Verification items for the finished model (mm, model axes). A direction names the side the tool comes from. Coordinates: 2 decimals unless noted, no trailing zeros. Write each loop counter-clockwise with the first axis right and the second up, starting at its lowest first coordinate (ties: lowest second). Pieces come first, ordered by that corner, then holes. Notation, with made-up numbers: (58, 48.5) -> (102, 48.5) arc R15 ccw to (102, 60.5) -> close; hole circle Ø4 at (20, 5.5). An arc over 180 degrees is marked (long way). Answer in a Markdown table with one row per item.
```python
from build123d import *

# Parameters (mm, degrees)
BOSS_EXTRUDE1_DEPTH = 10
SKETCH3_R           = 5
BOSS_EXTRUDE2_DEPTH = 5
SKETCH4_W           = 12.842437823
SKETCH4_H           = 1
CUT_EXTRUDE1_DEPTH  = 5
SKETCH5_R           = 3.418084762
BOSS_EXTRUDE3_DEPTH = 5
SKETCH6_W           = 9.346993936
SKETCH6_H           = 1
CUT_EXTRUDE2_DEPTH  = 5
SKETCH7_R           = 42.668113091
SKETCH7_R_2         = 32.812087574
BOSS_EXTRUDE4_DEPTH = 16
SKETCH8_R           = 10.204262611
CUT_EXTRUDE3_DEPTH  = 16
SKETCH9_R           = 41.320841223
SKETCH9_R_2         = 29.431774833
BOSS_EXTRUDE5_DEPTH = 16
SKETCH10_R          = 10.002103031
CUT_EXTRUDE4_DEPTH  = 16
SKETCH11_R          = 5.125485485
CUT_EXTRUDE5_DEPTH  = 16
SKETCH12_R          = 4.662079799
CUT_EXTRUDE6_DEPTH  = 16


with BuildPart() as part:
    # Sketch1 → Boss-Extrude1 (new body)
    with BuildSketch(Plane(origin=(0, 0, 0), x_dir=(1, 0, 0), z_dir=(0, 1, 0))):
        Polygon((0, 0), (0, 70), (-10, 70), (-10, -10), (70, -10), (70, 0), align=None)
    extrude(amount=BOSS_EXTRUDE1_DEPTH)

    # Sketch3 → Boss-Extrude2 (add)
    with BuildSketch(Plane.XY.offset(10)):
        with Locations((65, 5)):
            Circle(SKETCH3_R)
    extrude(amount=BOSS_EXTRUDE2_DEPTH)

    # Sketch4 → Cut-Extrude1 (cut)
    with BuildSketch(Plane.XY.offset(15)):
        with Locations((61.851491479, 5)):
            Rectangle(SKETCH4_W, SKETCH4_H)
    extrude(amount=-CUT_EXTRUDE1_DEPTH, mode=Mode.SUBTRACT)

    # Sketch5 → Boss-Extrude3 (add)
    with BuildSketch(Plane.ZY.offset(10)):
        with Locations(Location((-44.354632579, 5, 0), (0, 0, 180))):
            Circle(SKETCH5_R)
    extrude(amount=BOSS_EXTRUDE3_DEPTH)

    # Sketch6 → Cut-Extrude2 (cut)
    with BuildSketch(Plane.ZY.offset(15)):
        with Locations((-49.962828941, 2.5)):
            Rectangle(SKETCH6_W, SKETCH6_H)
    extrude(amount=-CUT_EXTRUDE2_DEPTH, mode=Mode.SUBTRACT)

    # Sketch7 → Boss-Extrude4 (add)
    with BuildSketch(Plane(origin=(0, 0, 0), x_dir=(-1, 0, 0), z_dir=(0, 0, -1))):
        with Locations((-70, 5)):
            Circle(SKETCH7_R)
        with Locations((-70, 5)):
            Circle(SKETCH7_R_2, mode=Mode.SUBTRACT)
    extrude(amount=-BOSS_EXTRUDE4_DEPTH)

    # Sketch8 → Cut-Extrude3 (cut)
    with BuildSketch(Plane(origin=(0, 0, 0), x_dir=(-1, 0, 0), z_dir=(0, 0, -1))):
        with Locations((-70, 5)):
            Circle(SKETCH8_R)
    extrude(amount=-CUT_EXTRUDE3_DEPTH, mode=Mode.SUBTRACT)

    # Sketch9 → Boss-Extrude5 (add)
    with BuildSketch(Plane(origin=(0, 0, 0), x_dir=(0, 0, -1), z_dir=(1, 0, 0))):
        with Locations((70, 5)):
            Circle(SKETCH9_R)
        with Locations((70, 5)):
            Circle(SKETCH9_R_2, mode=Mode.SUBTRACT)
    extrude(amount=-BOSS_EXTRUDE5_DEPTH)

    # Sketch10 → Cut-Extrude4 (cut)
    with BuildSketch(Plane(origin=(0, 0, 0), x_dir=(0, 0, -1), z_dir=(1, 0, 0))):
        with Locations((70, 5)):
            Circle(SKETCH10_R)
    extrude(amount=-CUT_EXTRUDE4_DEPTH, mode=Mode.SUBTRACT)

    # Sketch11 → Cut-Extrude5 (cut)
    with BuildSketch(Plane(origin=(0, 0, 0), x_dir=(0, 0, -1), z_dir=(1, 0, 0))):
        with Locations((70, 42.5)):
            Circle(SKETCH11_R)
    extrude(amount=-CUT_EXTRUDE5_DEPTH, mode=Mode.SUBTRACT)

    # Sketch12 → Cut-Extrude6 (cut)
    with BuildSketch(Plane(origin=(0, 0, 0), x_dir=(-1, 0, 0), z_dir=(0, 0, -1))):
        with Locations((-70, 42.5)):
            Circle(SKETCH12_R)
    extrude(amount=-CUT_EXTRUDE6_DEPTH, mode=Mode.SUBTRACT)


solid = part.part
```
1. Material ranges on probe 1 along Z at (x, y) = (-8.75, 5); probe 2 along Z at (x, y) = (38, -19.5); probe 3 along Y at (x, z) = (-7.75, -70), recorded low to high. Write a range as from..to.
Findings below:
| item | result |
|---|---|
| probe 1 | z = -111.32..-99.43, -60..10 |
| probe 2 | z = 0..16 |
| probe 3 | y = -36.32..-24.43, 34.43..37.37 |
2. Access from +Z, -Z, +X, -X, +Y, -Y to the whole of each face (thin tool, end or side, straight path). Record for faces 1 (the face through (49, 0, 5)), 2 (the face through (0, 2, -60)), 3 (the face through (-15, 5, -44)).
Findings below:
| item | result |
|---|---|
| face 1 | +Z, -Z |
| face 2 | -Z, +X, +Y, -Y |
| face 3 | -X |
3. Sectioned sample at C-C, the plane y = 5. Record the cut outline in (x, z).
Findings below:
| item | result |
|---|---|
| outline | (-16, -111.32) -> (0, -111.32) -> (0, -99.43) -> (-16, -99.43) -> close; (-16, -40.57) -> (-10, -40.57) -> (-10, -40.94) -> (-15, -40.94) -> (-15, -47.77) -> (-10, -47.77) -> (-10, -60) -> (0, -60) -> (0, 0) -> (59.8, 0) -> (59.8, 10) -> (37.19, 10) -> (37.19, 16) -> (27.33, 16) -> (27.33, 10) -> (-10, 10) -> (-10, -28.68) -> (-16, -28.68) -> close; (102.81, 0) -> (112.67, 0) -> (112.67, 16) -> (102.81, 16) -> close |
4. Sectioned sample at D-D, the plane z = -86. Record the cut outline in (x, y).
Findings below:
| item | result |
|---|---|
| outline | (-16, -33.1) -> (0, -33.1) -> (0, -19.7) -> (-16, -19.7) -> close; (-16, 29.7) -> (0, 29.7) -> (0, 43.1) -> (-16, 43.1) -> close |
5. Go/stop test with flat-tipped pins: pin 1 (7.5 mm diameter, centred on x = 70, y = 42.5, fed in from -Z); pin 2 (0.6 mm diameter, centred on x = -13.5, z = -46.5, fed in from -Y); pin 3 (5 mm diameter, centred on x = 48, z = 6.5, fed in from -Y); pin 4 (11 mm diameter, centred on x = 52.5, z = 6, fed in from +Y). Record where each tip stops, or that it passes through.
Findings below:
| item | result |
|---|---|
| pin 1 | passes through |
| pin 2 | stops at y = -29.19 |
| pin 3 | stops at y = -32.95 |
| pin 4 | stops at y = 45.95 |
6. Sectioned sample at A-A, the plane x = 70. Count the separate pieces of the cut face and the enclosed holes in it, and give its area (3 significant figures).
Findings below:
| item | result |
|---|---|
| separate pieces | 3 |
| enclosed holes | 0 |
| area | 166 mm² |
7. Sectioned sample at B-B, the plane y = -8. Record the cut outline in (x, z), and give its area (3 significant figures).
Findings below:
| item | result |
|---|---|
| outline | (-16, -109.22) -> (0, -109.22) -> (0, -96.41) -> (-16, -96.41) -> close; (-16, -43.59) -> (0, -43.59) -> (0, -30.78) -> (-16, -30.78) -> close; (29.36, 0) -> (39.87, 0) -> (39.87, 16) -> (29.36, 16) -> close; (100.13, 0) -> (110.64, 0) -> (110.64, 16) -> (100.13, 16) -> close |
| area | 747 mm² |
8. Release check for a two-part mould opening along Y. For faces 4 (the face through (-7.888, 37.377, -69.83)), 5 (the face through (-7.888, -36.283, -68.233)), 6 (the face through (-4, 10, -1)), 7 (the face through (-12.46, 7.47, -41.99)) record: released by +Y, released by -Y, zero draft, split by the parting line, or undercut.
Findings below:
| item | result |
|---|---|
| face 4 | undercut |
| face 5 | split by the parting line |
| face 6 | released by +Y |
| face 7 | undercut |
